from build123d import *

# Parameters (mm, degrees)
SKETCH1_R           = 1.7
SKETCH1_R_2         = 2.1
BOSS_EXTRUDE1_DEPTH = 8.5
SKETCH2_R           = 2.15
CUT_EXTRUDE1_DEPTH  = 8.2
CUT_EXTRUDE3_DEPTH  = 4.5


# Read off the part's stored shape, not the designer's step: AdvancedHole1
with BuildPart() as part:
    # Sketch1 → Boss-Extrude1 (new body)
    with BuildSketch(Plane.XY):
        with BuildLine():
            Line((-16.436457619, 29), (-11.155935204, 29))
            ThreePointArc((-11.155935204, 29), (-9.748616749, 29.926511277), (-9.214880919, 31.524664725))
            ThreePointArc((-9.214880919, 31.524664725), (0, 40.739545643), (9.214880919, 31.524664725))
            ThreePointArc((9.214880919, 31.524664725), (9.748616749, 29.926511277), (11.155935204, 29))
            Line((11.155935204, 29), (17.063542381, 29))
            Line((17.063542381, 29), (17.063542381, -29))
            Line((17.063542381, -29), (11.155935204, -29))
            ThreePointArc((11.155935204, -29), (9.748616749, -29.926511277), (9.214880919, -31.524664725))
            ThreePointArc((9.214880919, -31.524664725), (0, -40.739545643), (-9.214880919, -31.524664725))
            ThreePointArc((-9.214880919, -31.524664725), (-9.748616749, -29.926511277), (-11.155935204, -29))
            Line((-11.155935204, -29), (-16.436457619, -29))
            Line((-16.436457619, -29), (-16.436457619, 29))
        make_face()
        with Locations((-13.5, 25.3)):
            Circle(SKETCH1_R, mode=Mode.SUBTRACT)
        with Locations((13.5, -25.3)):
            Circle(SKETCH1_R, mode=Mode.SUBTRACT)
        with Locations((-13.5, -25.3)):
            Circle(SKETCH1_R, mode=Mode.SUBTRACT)
        with Locations((13.5, 25.3)):
            Circle(SKETCH1_R, mode=Mode.SUBTRACT)
        with Locations((0, 35)):
            Circle(SKETCH1_R_2, mode=Mode.SUBTRACT)
        with Locations(Location((0, -35, 0), (0, 0, 180))):
            Circle(SKETCH1_R_2, mode=Mode.SUBTRACT)
        with BuildLine():
            Line((-13.5, 16), (13.5, 16))
            Line((13.5, 16), (13.5, -16))
            Line((13.5, -16), (2.3, -16))
            ThreePointArc((2.3, -16), (1.678013477, -15.060993262), (1.3, -14))
            ThreePointArc((1.3, -14), (0.921986523, -15.060993262), (0.3, -16))
            Line((0.3, -16), (-13.5, -16))
            Line((-13.5, -16), (-13.5, 16))
        make_face(mode=Mode.SUBTRACT)
    extrude(amount=BOSS_EXTRUDE1_DEPTH)

    # Sketch2 → Cut-Extrude1 (cut)
    with BuildSketch(Plane.XY.offset(8.5)):
        with Locations((-12, 20)):
            Circle(SKETCH2_R)
        with Locations((-6, 20)):
            Circle(SKETCH2_R)
        with Locations((0, 20)):
            Circle(SKETCH2_R)
        with Locations((6, 20)):
            Circle(SKETCH2_R)
        with Locations((12, 20)):
            Circle(SKETCH2_R)
        with Locations((-6, 26)):
            Circle(SKETCH2_R)
        with Locations((0, 26)):
            Circle(SKETCH2_R)
        with Locations((6, 26)):
            Circle(SKETCH2_R)
        with Locations((-11.967349369, -20)):
            Circle(SKETCH2_R)
        with Locations((-5.983674685, -20)):
            Circle(SKETCH2_R)
        with Locations((0, -20)):
            Circle(SKETCH2_R)
        with Locations((5.983674685, -20)):
            Circle(SKETCH2_R)
        with Locations((11.967349369, -20)):
            Circle(SKETCH2_R)
        with Locations((-5.983674685, -26)):
            Circle(SKETCH2_R)
        with Locations((0, -26)):
            Circle(SKETCH2_R)
        with Locations((5.983674685, -26)):
            Circle(SKETCH2_R)
    extrude(amount=-CUT_EXTRUDE1_DEPTH, mode=Mode.SUBTRACT)

    # AdvancedHole1 outline → AdvancedHole1 (revolve, cut)
    with BuildSketch(Plane(origin=(-13.5, -25.3, 0), x_dir=(1, 0, 0), z_dir=(0, -1, 0))):
        Polygon((3.47, 0), (1.7, 1.77), (1.7, 0), align=None)
    revolve(axis=Axis((-13.5, -25.3, 0), (0, 0, 1)), mode=Mode.SUBTRACT)

    # AdvancedHole1 2 outline → AdvancedHole1 2 (revolve, cut)
    with BuildSketch(Plane(origin=(13.5, -25.3, 0), x_dir=(1, 0, 0), z_dir=(0, -1, 0))):
        Polygon((3.47, 0), (1.7, 1.77), (1.7, 0), align=None)
    revolve(axis=Axis((13.5, -25.3, 0), (0, 0, 1)), mode=Mode.SUBTRACT)

    # AdvancedHole1 3 outline → AdvancedHole1 3 (revolve, cut)
    with BuildSketch(Plane(origin=(-13.5, 25.3, 0), x_dir=(1, 0, 0), z_dir=(0, -1, 0))):
        Polygon((3.47, 0), (1.7, 1.77), (1.7, 0), align=None)
    revolve(axis=Axis((-13.5, 25.3, 0), (0, 0, 1)), mode=Mode.SUBTRACT)

    # AdvancedHole1 4 outline → AdvancedHole1 4 (revolve, cut)
    with BuildSketch(Plane(origin=(13.5, 25.3, 0), x_dir=(1, 0, 0), z_dir=(0, -1, 0))):
        Polygon((3.47, 0), (1.7, 1.77), (1.7, 0), align=None)
    revolve(axis=Axis((13.5, 25.3, 0), (0, 0, 1)), mode=Mode.SUBTRACT)

    # Sketch6 → Cut-Extrude3 (cut)
    with BuildSketch(Plane.XY.offset(8.5)):
        Polygon((-9.144659307, 29.348390155), (9.144659307, 29.348390155), (9.144659307, 23.081210136), (15.140663267, 23.081210136), (15.140663267, 16.512723385), (-15.140663267, 16.512723385), (-15.140663267, 23.081210136), (-9.144659307, 23.081210136), align=None)
        Polygon((-9.144659307, -23.081210136), (-15.140663267, -23.081210136), (-15.140663267, -16.512723385), (15.140663267, -16.512723385), (15.140663267, -23.081210136), (9.144659307, -23.081210136), (9.144659307, -29.348390155), (-9.144659307, -29.348390155), align=None)
    extrude(amount=-CUT_EXTRUDE3_DEPTH, mode=Mode.SUBTRACT)


solid = part.part
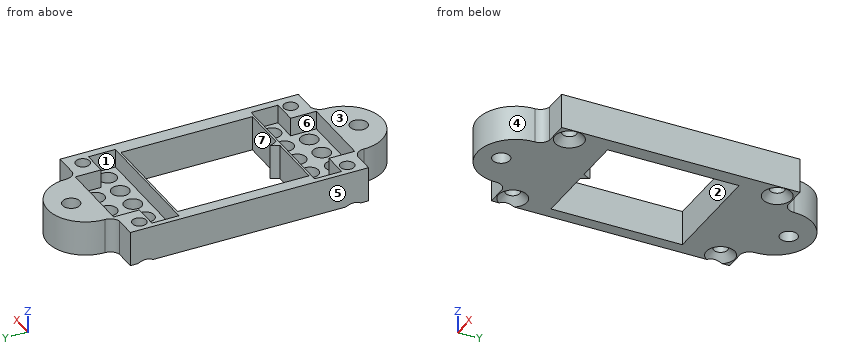
Here's how the part is built. I have some questions about the finished solid (model axes, mm). Face numbers are marked on the shaded views. A direction names the side the tool comes from. Coordinates: 2 decimals unless noted, no trailing zeros. Write each loop counter-clockwise with the first axis right and the second up, starting at its lowest first coordinate (ties: lowest second). Pieces come first, ordered by that corner, then holes. Notation, with made-up numbers: (7, -10.5) - (45, -10.5) arc R14 ccw to (45, 15.5) - close; hole circle Ø10 at (55, -25.75). An arc over 180 degrees is marked (long way). Use one line per item in the form item = value.
1) Suppose I cut it at D-D, the plane y = -20. Write out the boundary of the cut face in (x, z).
Solved:
outline = (-16.44, 0) - (17.06, 0) - (17.06, 8.5) - (15.14, 8.5) - (15.14, 4) - (14.12, 4) - (14.12, 0.3) - (9.82, 0.3) - (9.82, 4) - (8.13, 4) - (8.13, 0.3) - (3.83, 0.3) - (3.83, 4) - (2.15, 4) - (2.15, 0.3) - (-2.15, 0.3) - (-2.15, 4) - (-3.83, 4) - (-3.83, 0.3) - (-8.13, 0.3) - (-8.13, 4) - (-9.82, 4) - (-9.82, 0.3) - (-14.12, 0.3) - (-14.12, 4) - (-15.14, 4) - (-15.14, 8.5) - (-16.44, 8.5) - close
2) Thinking about a two-plate mould opening in X: for the marked faces 4, 5, 6 and 7, which applies, released by +X, released by -X, zero draft, split by the parting line, or undercut?
Solved:
face_4 = split by the parting line
face_5 = released by -X
face_6 = undercut
face_7 = undercut
3) Suppose I cut it at A-A, the plane y = 2. Write out the boundary of the cut face in (x, z), plus the area to 4 significant figures.
Solved:
outline = (-16.44, 0) - (-13.5, 0) - (-13.5, 8.5) - (-16.44, 8.5) - close; (13.5, 0) - (17.06, 0) - (17.06, 8.5) - (13.5, 8.5) - close
area = 55.25 mm2
4) I need wall thicknesses on line 1 (X direction, y = -23, z = 5); line 2 (X direction, y = 2.5, z = 6); line 3 (Y direction, x = -5, z = 7). Which ranges of each line are inside material? Lowest first, please.
Solved:
line_1 = -16.44 to -15.14, 15.14 to 17.06
line_2 = -16.44 to -13.5, 13.5 to 17.06
line_3 = -39.27 to -29.35, -16.51 to -16, 16 to 16.51, 29.35 to 39.27
5) On a 3-axis mill with a long thin cutter (end or side, diameter ignored), from which of +Z, -Z, +X, -X, +Y, -Y can I reach the whole of each face in a straight line? I mean the marked faces 1, 2 and 3. Say none if no direction works.
Solved:
face_1 = +Z
face_2 = +Z, -Z
face_3 = +Z, +X, -X, +Y, -Y
6) I'm going to push flat-ended pins straight in: P1, Ø4, axis at x = 0, y = 26, coming from the -Z side; P2, Ø3.5, axis at x = 11.5, y = -20, coming from the +Z side; P3, Ø1.3, axis at x = 6, y = -26, coming from the +Z side; P4, Ø5, axis at x = -12, z = 6.5, coming from the +Y side. Where does each tip first touch, or does it pass through?
Solved:
P1 = 0
P2 = 4
P3 = 0.3
P4 = 30.32
7) Suppose I cut it at C-C, the plane z = 7.75. Give the number of separate pieces and of enclosed holes in the cut face, plus the area to 3 significant figures.
Solved:
separate_pieces = 1
enclosed_holes = 9
area = 754 mm2
